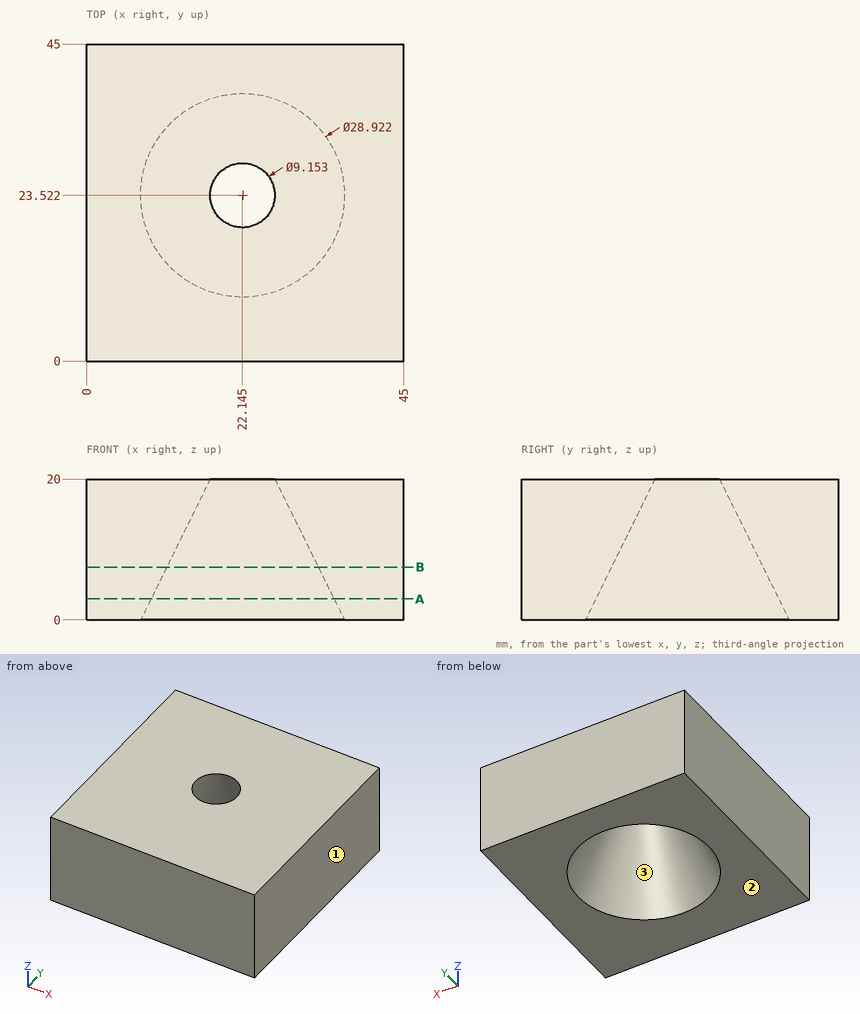
Geometry check sheet. Reference: drawing and pictorial views, mm from the part's lowest x, y, z. Coordinates: 2 decimals unless noted, no trailing zeros. Write each loop counter-clockwise with the first axis right and the second up, starting at its lowest first coordinate (ties: lowest second). Pieces come first, ordered by that corner, then holes. Notation, with made-up numbers: (78.25, 11) -> (104.25, 11) arc R26 ccw to (104.25, 38) -> close; hole circle Ø1 at (19.5, 7.25). An arc over 180 degrees is marked (long way). One line per question, with ' | ' between items.
1. Cross-section at B-B on z = 7.5. Record the cut outline in (x, y) (1 decimal), and give its area (3 significant figures).
Answers:
outline: (0, 0) -> (45, 0) -> (45, 45) -> (0, 45) -> close; hole circle Ø21.5 at (22.1, 23.5) | area: 1,660 mm²
2. Thickness scan on probe 1 along X at (y, z) = (19, 5); probe 2 along Y at (x, z) = (17.5, 4.5); probe 3 along Y at (x, z) = (33, 3.5) (1 decimal). Record the ranges inside material, lowest first. Write a range as from..to.
Answers:
probe 1: x = 0..11.04, 33.25..45 | probe 2: y = 0..12.2, 34.84..45 | probe 3: y = 0..16.9, 30.2..45
3. Draft check along X on the marked faces 1, 2 and 3. Enter one of: +X half, -X half, draft (parallel to the pull), parting line (faces both ways), or undercut.
Answers:
face 1: +X half | face 2: draft | face 3: undercut
4. Cross-section at A-A on z = 3. Record the cut outline in (x, y) (1 decimal).
Answers:
outline: (0, 0) -> (45, 0) -> (45, 45) -> (0, 45) -> close; hole circle Ø26 at (22.1, 23.5)
